Geometry check sheet. Reference: drawing and pictorial views, mm from the part's lowest x, y, z. A direction names the side the tool comes from. Give positions to 0.01 mm unless a question says otherwise; leave off trailing zeros. Loops run counter-clockwise (first coordinate to the right, second up) from the corner with the lowest first, then second, coordinate; pieces in that order, holes last. Notation, with made-up numbers: (77.5, 61) - (86.5, 61) arc R17 ccw to (86.5, 88) - close; hole circle Ø5 at (54.25, 22). An arc over 180 degrees is marked (long way). One line per question, with ' | ' between items. Start each with the question number.
1. Section check C-C, the plane z = 14. Enter the section's corners in (x, y), then the cut area to 3 significant figures.
2. Mould release check, pull along X, two halves, no side actions. Record for the marked faces 3, 4 and 5: +X half, -X half, draft (parallel to the pull), parting line (faces both ways), or undercut.
3. Section check A-A, the plane z = 6.5. Enter the section's corners in (x, y), then the cut area to 3 significant figures.
4. Thickness scan on line 1 along Z through (x, y) = (2, 2.75); line 2 along X through (y, z) = (4, 13.25); line 3 along X through (y, z) = (2.25, 13). Record the ranges inside material, lowest first. Write a range as from..to.
5. Section check B-B, the plane y = 2.5. Enter the section's corners in (x, z), then the cut area to 3 significant figures.
6. Tool access check on the marked faces 1 and 2. Record the directions out of +Z, -Z, +X, -X, +Y, -Y that give a thin tool (end or side, any length) a straight path to the whole face; none if there is none.
7. Section check D-D, the plane x = 2.5. Enter the section's corners in (y, z), then the cut area to 3 significant figures.
8. Depth check by flat-ended pin: pin 1 Ø2.5 at (x, y) = (3, 3.46) entering from -Z; pin 2 Ø1 at (x, z) = (2, 10.5) entering from +Y; pin 3 Ø1.5 at (x, y) = (3.5, 3) entering from +Z. Enter the tip coordinate at first touch or a pass-through.
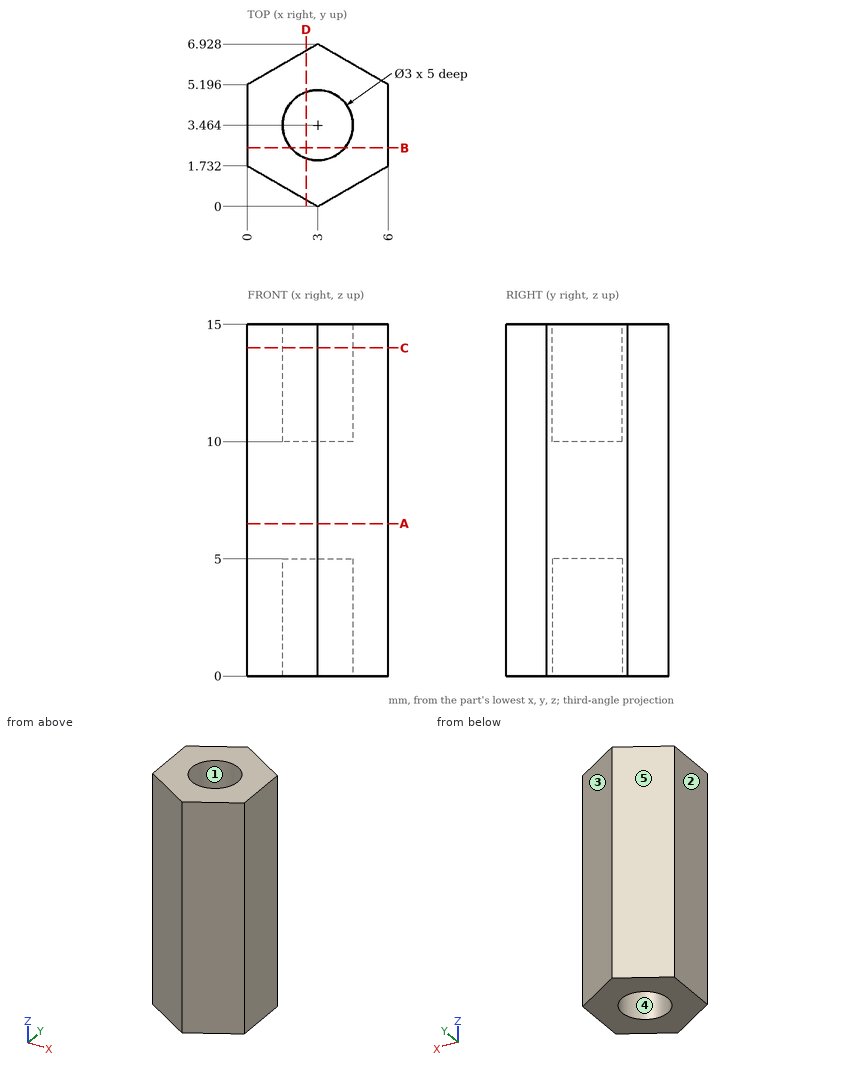
Results list:
1) outline: (0, 1.73) - (3, 0) - (6, 1.73) - (6, 5.2) - (3, 6.93) - (0, 5.2) - close; hole circle Ø3 at (3, 3.46) | area: 24.1 mm²
2) face 3: +X half | face 4: undercut | face 5: -X half
3) outline: (0, 1.73) - (3, 0) - (6, 1.73) - (6, 5.2) - (3, 6.93) - (0, 5.2) - close | area: 31.2 mm²
4) line 1: 5..10 | line 2: 0..1.6, 4.4..6 | line 3: 0..2.12, 3.88..6
5) outline: (0, 0) - (1.85, 0) - (1.85, 5) - (4.15, 5) - (4.15, 0) - (6, 0) - (6, 15) - (4.15, 15) - (4.15, 10) - (1.85, 10) - (1.85, 15) - (0, 15) - close | area: 67.0 mm²
6) face 1: +Z | face 2: +Z, -Z, -X, +Y, -Y
7) outline: (0.29, 0) - (2.05, 0) - (2.05, 5) - (4.88, 5) - (4.88, 0) - (6.64, 0) - (6.64, 15) - (4.88, 15) - (4.88, 10) - (2.05, 10) - (2.05, 15) - (0.29, 15) - close | area: 67.0 mm²
8) pin 1: z = 5 | pin 2: y = 6.64 | pin 3: z = 10
